For this review, take the finished solid that the model builds, in its own axes (mm). Face numbers are marked on the shaded views. Round coordinates to 2 decimals unless told otherwise and drop trailing zeros. Loops run counter-clockwise (first coordinate to the right, second up) from the corner with the lowest first, then second, coordinate; pieces in that order, holes last.
1) Take a section at C-C (x = 66). State the section outline as (y, z) points.
2) Wall thickness on L1, parallel to X at y = 1.1, z = 41.6; L2, parallel to X at y = 0.8, z = -33.4; L3, parallel to X at y = 1.3, z = 36.28: over which ranges is each line inside the solid? List them lowest first.
3) Take a section at B-B (z = -10.5). State the section outline as (x, y) points.
4) Mouldability with a two-part tool opening along Y and no side actions: class the marked faces 1 and 2 as pulls with the +Y half, pulls with the -Y half, needs draft (parallel to the pull), parting line crosses it, or undercut.
5) Take a section at D-D (y = 2.1). Give the number of separate pieces and of enclosed holes in the cut face, then the cut area to 3 significant figures.
6) Insertion check: pin 1 (4 mm diameter, centred on x = -17.5, z = 41.6, fed in from +Y); pin 2 (0.9 mm diameter, centred on x = 63, y = 2, fed in from -Z); pin 3 (1.5 mm diameter, centred on y = 1.5, z = -88, fed in from +X); pin 4 (0.9 mm diameter, centred on y = 2, z = -13.5, fed in from -X). Each pin has a flat end and moves straight along its axis. Give the tip position at first contact, or say it passes through.
7) Take a section at A-A (x = 7). State the section outline as (y, z) points.
```python
from build123d import *

# Parameters (mm, degrees)
BODY_DEPTH              = 3
SKETCH4_R               = 1.55
MOTOR_MOUNT_DEPTH       = 3
SKETCH5_R               = 1.1
SKETCH5_W               = 25.4
SKETCH5_H               = 42
PROTOBOARD_MOUNT_DEPTH  = 10
SKETCH8_R               = 1.55
STAND_OFF_MOUNT_DEPTH   = 10
SKETCH9_W               = 30
SKETCH9_H               = 35
BOSS_EXTRUDE1_DEPTH     = 3
SKETCH10_R              = 1.55
CUT_EXTRUDE1_DEPTH      = 164.321768298
SKETCH11_R              = 1.55
CASTER_BALL_MOUNT_DEPTH = 164.321768298


with BuildPart() as part:
    # Sketch3 → Body (new body)
    with BuildSketch(Plane(origin=(0, 0, 0), x_dir=(1, 0, 0), z_dir=(0, 1, 0))):
        Polygon((-15, -46), (-47, -46), (-47, 34), (-20, 144), (20, 144), (47, 34), (47, -46), (15, -46), (15, 0), (-15, 0), align=None)
    extrude(amount=BODY_DEPTH)

    # Sketch4 → Motor Mount (cut)
    with BuildSketch(Plane(origin=(0, 3, 0), x_dir=(1, 0, 0), z_dir=(0, 1, 0))):
        with Locations(Location((-18.29, -3.65, 0), (0, 0, 270))):
            Circle(SKETCH4_R)
        with Locations(Location((18.29, -3.65, 0), (0, 0, 90))):
            Circle(SKETCH4_R)
        with Locations(Location((-18.29, 39.53, 0), (0, 0, 270))):
            Circle(SKETCH4_R)
        with Locations(Location((18.29, 39.53, 0), (0, 0, 270))):
            Circle(SKETCH4_R)
    extrude(amount=-MOTOR_MOUNT_DEPTH, mode=Mode.SUBTRACT)

    # Sketch5 → Protoboard Mount (cut)
    with BuildSketch(Plane(origin=(0, 3, 0), x_dir=(1, 0, 0), z_dir=(0, 1, 0))):
        with Locations(Location((-17.8, 103.5, 0), (0, 0, 270))):
            Circle(SKETCH5_R)
        with Locations(Location((17.8, 103.5, 0), (0, 0, 270))):
            Circle(SKETCH5_R)
        with Locations((0, 81)):
            Rectangle(SKETCH5_W, SKETCH5_H)
    extrude(amount=-PROTOBOARD_MOUNT_DEPTH, mode=Mode.SUBTRACT)

    # Sketch8 → Stand Off Mount (cut)
    with BuildSketch(Plane(origin=(0, 3, 0), x_dir=(1, 0, 0), z_dir=(0, 1, 0))):
        with Locations(Location((-22.5, 88.4, 0), (0, 0, 270))):
            Circle(SKETCH8_R)
        with Locations(Location((22.5, 88.4, 0), (0, 0, 270))):
            Circle(SKETCH8_R)
        with Locations(Location((37.5, 33.4, 0), (0, 0, 270))):
            Circle(SKETCH8_R)
        with Locations(Location((-37.5, 33.4, 0), (0, 0, 270))):
            Circle(SKETCH8_R)
        with Locations(Location((-17.5, -41.6, 0), (0, 0, 270))):
            Circle(SKETCH8_R)
        with Locations(Location((17.5, -41.6, 0), (0, 0, 270))):
            Circle(SKETCH8_R)
    extrude(amount=-STAND_OFF_MOUNT_DEPTH, mode=Mode.SUBTRACT)

    # Sketch9 → Boss-Extrude1 (add)
    with BuildSketch(Plane(origin=(0, 3, 0), x_dir=(1, 0, 0), z_dir=(0, 1, 0))):
        with Locations((62, -28.5)):
            Rectangle(SKETCH9_W, SKETCH9_H)
        with Locations((-62, -28.5)):
            Rectangle(SKETCH9_W, SKETCH9_H)
    extrude(amount=-BOSS_EXTRUDE1_DEPTH)

    # Sketch10 → Cut-Extrude1 (cut, through all)
    with BuildSketch(Plane(origin=(0, 3, 0), x_dir=(1, 0, 0), z_dir=(0, 1, 0))):
        with Locations(Location((-52.2, -20.72, 0), (0, 0, 270))):
            Circle(SKETCH10_R)
        with Locations(Location((-32.2, -20.72, 0), (0, 0, 270))):
            Circle(SKETCH10_R)
        with Locations(Location((-52.2, -36.28, 0), (0, 0, 270))):
            Circle(SKETCH10_R)
        with Locations(Location((-32.2, -36.28, 0), (0, 0, 270))):
            Circle(SKETCH10_R)
        with Locations(Location((32.2, -36.28, 0), (0, 0, 90))):
            Circle(SKETCH10_R)
        with Locations(Location((52.2, -36.28, 0), (0, 0, 90))):
            Circle(SKETCH10_R)
        with Locations(Location((32.2, -20.72, 0), (0, 0, 90))):
            Circle(SKETCH10_R)
        with Locations(Location((52.2, -20.72, 0), (0, 0, 90))):
            Circle(SKETCH10_R)
    extrude(amount=-CUT_EXTRUDE1_DEPTH, mode=Mode.SUBTRACT)

    # Sketch11 → Caster Ball Mount (cut, through all)
    with BuildSketch(Plane(origin=(0, 3, 0), x_dir=(1, 0, 0), z_dir=(0, 1, 0))):
        with Locations(Location((-23, 96.4, 0), (0, 0, 270))):
            Circle(SKETCH11_R)
        with Locations(Location((-23, 106.4, 0), (0, 0, 270))):
            Circle(SKETCH11_R)
        with Locations(Location((-23, 116.4, 0), (0, 0, 270))):
            Circle(SKETCH11_R)
        with Locations(Location((23, 96.4, 0), (0, 0, 90))):
            Circle(SKETCH11_R)
        with Locations(Location((23, 106.4, 0), (0, 0, 90))):
            Circle(SKETCH11_R)
        with Locations(Location((23, 116.4, 0), (0, 0, 90))):
            Circle(SKETCH11_R)
    extrude(amount=-CASTER_BALL_MOUNT_DEPTH, mode=Mode.SUBTRACT)


solid = part.part
```
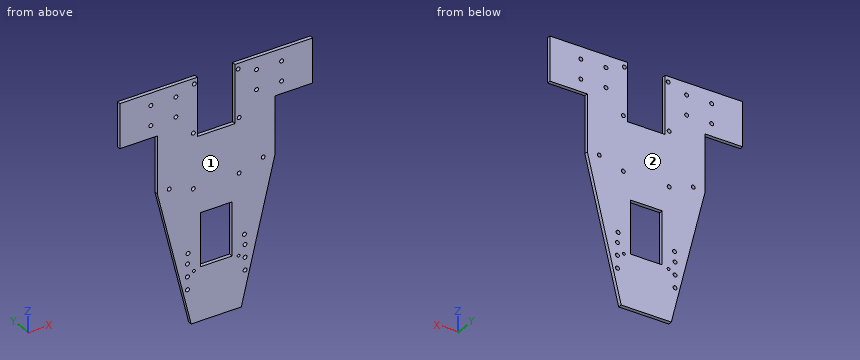
Response:
1. outline: (0, 11) - (3, 11) - (3, 46) - (0, 46) - close
2. L1: x = -77 to -19.05, -15.95 to -15, 15 to 15.95, 19.05 to 77
2. L2: x = -47 to -39.05, -35.95 to 35.95, 39.05 to 47
2. L3: x = -77 to -53.75, -50.65 to -33.75, -30.65 to -15, 15 to 30.65, 33.75 to 50.65, 53.75 to 77
3. outline: (-47, 0) - (47, 0) - (47, 3) - (-47, 3) - close
4. face 1: pulls with the -Y half
4. face 2: pulls with the +Y half
5. separate pieces: 1
5. enclosed holes: 27
5. area: 14,400 mm2
6. pin 1: stops at y = 3
6. pin 2: stops at z = 11
6. pin 3: stops at x = 33.93
6. pin 4: stops at x = -47
7. outline: (0, -144) - (3, -144) - (3, -102) - (0, -102) - close; (0, -60) - (3, -60) - (3, 0) - (0, 0) - close
